from build123d import *

# Parameters (mm, degrees)
BOSS_EXTRUDE1_DEPTH = 6
FILLET1_R           = 10
SKETCH2_W           = 5
SKETCH2_H           = 9.5
SKETCH2_W_2         = 10
SKETCH2_H_2         = 11
CUT_EXTRUDE1_DEPTH  = 60.571910327
CHAMFER1_SIZE       = 8.75


with BuildPart() as part:
    # Sketch1 → Boss-Extrude1 (new body)
    with BuildSketch(Plane.XY):
        Polygon((0, 0), (42.3, 0), (42.3, 15.15), (57.3, 15.15), (57.3, -15), (-15, -15), (-15, 15.15), (0, 15.15), align=None)
    extrude(amount=BOSS_EXTRUDE1_DEPTH)

    # Fillet1
    fillet1_edges = [part.edges().sort_by_distance(p)[0] for p in [
        (57.3, -15, 3),
        (-15, -15, 3),
    ]]
    fillet(fillet1_edges, radius=FILLET1_R)

    # Sketch2 → Cut-Extrude1 (cut, through all)
    with BuildSketch(Plane(origin=(0, 0, 0), x_dir=(-1, 0, 0), z_dir=(0, 0, -1))):
        with Locations((-49.8, 10.4)):
            Rectangle(SKETCH2_W, SKETCH2_H)
        with Locations((-49.8, 0.15)):
            Rectangle(SKETCH2_W_2, SKETCH2_H_2)
    cut_extrude1 = extrude(amount=-CUT_EXTRUDE1_DEPTH, mode=Mode.SUBTRACT)

    # Mirror1: Cut-Extrude1 across plane
    add(cut_extrude1.mirror(Plane(origin=(21.15, 0, 0), x_dir=(0, 0, 1), z_dir=(1, 0, 0))), mode=Mode.SUBTRACT)

    # Chamfer1
    chamfer1_edges = [part.edges().sort_by_distance(p)[0] for p in [
        (0, 0, 3),
        (42.3, 0, 3),
    ]]
    chamfer(chamfer1_edges, length=CHAMFER1_SIZE)


solid = part.part
Verification items for the finished model (mm, model axes). A direction names the side the tool comes from. Coordinates: 2 decimals unless noted, no trailing zeros. Write each loop counter-clockwise with the first axis right and the second up, starting at its lowest first coordinate (ties: lowest second). Pieces come first, ordered by that corner, then holes. Notation, with made-up numbers: (81, 89.25) -> (109, 89.25) arc R26 ccw to (109, 118.25) -> close; hole circle Ø4 at (31.25, -24.75). An arc over 180 degrees is marked (long way). One line per item, written item: value. Start each with the question number.
Q1. Access from +Z, -Z, +X, -X, +Y, -Y to the whole of each face (thin tool, end or side, straight path). Record for faces 4 (the flat face through (57.3, 5, 3)), 5 (the flat face through (-4, 5.65, 3)), 6 (the flat face through (52.3, 10, 3)).
Q2. Cross-section at B-B on y = 5. Enter the section's corners in (x, z).
Q3. Cross-section at C-C on z = 4.75. Enter the section's corners in (x, y), and give its area (3 significant figures).
Q4. Cross-section at A-A on y = -2.5. Enter the section's corners in (x, z).
Q5. Cross-section at D-D on x = 2. Enter the section's corners in (y, z).
Q6. Go/stop test with flat-tipped pins: P1, Ø3, axis at x = 19, z = 3.5, coming from the +Y side; P2, Ø3, axis at x = 49, z = 2.5, coming from the +Y side; P3, Ø10, axis at x = 12.5, y = 2.5, coming from the -Z side; P4, Ø3, axis at x = -12, z = 3.5, coming from the -Y side. Record where each tip stops, or that it passes through.
Q7. Mould release check, pull along Y, two halves, no side actions. Record for faces 1 (the flat face through (-10, 10, 3)), 2 (the flat face through (-13, 15.15, 3)), 3 (the flat face through (50, -5.35, 3)): pulls with the +Y half, pulls with the -Y half, needs draft (parallel to the pull), parting line crosses it, or undercut.
Q8. Thickness scan on L1, parallel to X at y = 14, z = 5.25; L2, parallel to X at y = -1.5, z = 3.25; L3, parallel to X at y = 0.5, z = 5. Record the ranges inside material, lowest first. Write a range as from..to.
Checked values:
1. face 4: +Z, -Z, +X, +Y, -Y
1. face 5: +Z, -Z
1. face 6: +Z, -Z, +Y
2. outline: (-15, 0) -> (-12.5, 0) -> (-12.5, 6) -> (-15, 6) -> close; (-2.5, 0) -> (3.75, 0) -> (3.75, 6) -> (-2.5, 6) -> close; (38.55, 0) -> (44.8, 0) -> (44.8, 6) -> (38.55, 6) -> close; (54.8, 0) -> (57.3, 0) -> (57.3, 6) -> (54.8, 6) -> close
3. outline: (-15, -5) arc R10 ccw to (-5, -15) -> (47.3, -15) arc R10 ccw to (57.3, -5) -> (57.3, 15.15) -> (52.3, 15.15) -> (52.3, 5.65) -> (54.8, 5.65) -> (54.8, -5.35) -> (44.8, -5.35) -> (44.8, 5.65) -> (47.3, 5.65) -> (47.3, 15.15) -> (42.3, 15.15) -> (42.3, 8.75) -> (33.55, 0) -> (8.75, 0) -> (0, 8.75) -> (0, 15.15) -> (-5, 15.15) -> (-5, 5.65) -> (-2.5, 5.65) -> (-2.5, -5.35) -> (-12.5, -5.35) -> (-12.5, 5.65) -> (-10, 5.65) -> (-10, 15.15) -> (-15, 15.15) -> close
3. area: 1,260 mm²
4. outline: (-15, 0) -> (-12.5, 0) -> (-12.5, 6) -> (-15, 6) -> close; (-2.5, 0) -> (44.8, 0) -> (44.8, 6) -> (-2.5, 6) -> close; (54.8, 0) -> (57.3, 0) -> (57.3, 6) -> (54.8, 6) -> close
5. outline: (-15, 0) -> (6.75, 0) -> (6.75, 6) -> (-15, 6) -> close
6. P1: stops at y = 0
6. P2: stops at y = -5.35
6. P3: stops at z = 0
6. P4: stops at y = -13.35
7. face 1: needs draft
7. face 2: pulls with the +Y half
7. face 3: undercut
8. L1: x = -15..-10, -5..0, 42.3..47.3, 52.3..57.3
8. L2: x = -15..-12.5, -2.5..44.8, 54.8..57.3
8. L3: x = -15..-12.5, -2.5..8.25, 34.05..44.8, 54.8..57.3
